Verification items for the finished model (mm, model axes). A direction names the side the tool comes from. Give positions to 0.01 mm unless a question says otherwise; leave off trailing zeros. Order: outer loops, then holes, each group sorted by start corner. A loop starts at its lowest first (then second) coordinate and runs counter-clockwise, first axis right, second up.
from build123d import *

# Parameters (mm, degrees)
BOSS_EXTRUDE2_DEPTH = 50.25
SKETCH3_W           = 2
SKETCH3_H           = 1
CUT_EXTRUDE2_DEPTH  = 101.5
SKETCH4_W           = 4
SKETCH4_H           = 2
BOSS_EXTRUDE3_DEPTH = 5
CUT_EXTRUDE3_DEPTH  = 5.2


with BuildPart() as part:
    # LED Segment → Boss-Extrude2 (new body, symmetric)
    with BuildSketch(Plane(origin=(0, 0, 0), x_dir=(0, 0, -1), z_dir=(1, 0, 0))):
        Polygon((8.982863896, -5.225833025), (12, 0), (6, 10.392304845), (-6, 10.392304845), (-12, 0), (-8.982863896, -5.225833025), (-4.7, 2.192304845), (-4.7, 2.792304845), (-6.1, 4.192304845), (-6.1, 4.792304845), (-5.1, 4.792304845), (-5.1, 5.392304845), (5.1, 5.392304845), (5.1, 4.792304845), (6.1, 4.792304845), (6.1, 4.192304845), (4.7, 2.792304845), (4.7, 2.192304845), align=None)
    extrude(amount=BOSS_EXTRUDE2_DEPTH, both=True)

    # Sketch3 → Cut-Extrude2 (cut, through all)
    with BuildSketch(Plane(origin=(50.25, 0, 0), x_dir=(0, 0, -1), z_dir=(1, 0, 0))):
        with Locations((4, 9.892304845)):
            Rectangle(SKETCH3_W, SKETCH3_H)
        Polygon((10.5, -2.598076211), (11.5, -0.866025404), (10.633974596, -0.366025404), (9.633974596, -2.098076211), align=None)
    extrude(amount=-CUT_EXTRUDE2_DEPTH, mode=Mode.SUBTRACT)

    # Sketch4 → Boss-Extrude3 (add)
    with BuildSketch(Plane(origin=(50.25, 0, 0), x_dir=(0, 0, -1), z_dir=(1, 0, 0))):
        with Locations((0, 9.392304845)):
            Rectangle(SKETCH4_W, SKETCH4_H)
    extrude(amount=BOSS_EXTRUDE3_DEPTH)

    # Sketch5 → Cut-Extrude3 (cut)
    with BuildSketch(Plane.ZY.offset(50.25)):
        Polygon((-2.2, 10.392304845), (-2.2, 8.192304845), (2.2, 8.192304845), (2.2, 10.392304845), (2, 10.392304845), (-2, 10.392304845), align=None)
    extrude(amount=-CUT_EXTRUDE3_DEPTH, mode=Mode.SUBTRACT)


solid = part.part
(1) Set-up check for faces 5 (the flat face through (53, 9, 2)), 6 (the flat face through (-48, 9, 2.2)), 7 (the flat face through (0.7, -1.46, -6.81)): record each of +Z, -Z, +X, -X, +Y, -Y from which the full face is reachable in a straight line by a thin tool's end or side.
Solved:
face 5: +Z, +X, +Y, -Y
face 6: -X, +Y
face 7: +X, -X, -Y
(2) Go/stop test with flat-tipped pins: pin 1 (1 mm diameter, centred on x = 39, y = -2, fed in from +Z); pin 2 (4 mm diameter, centred on y = 8.5, z = 8, fed in from +X); pin 3 (0.7 mm diameter, centred on x = -7, y = 4.5, fed in from -Z). Record where each tip stops, or that it passes through.
Solved:
pin 1: stops at z = 11.13
pin 2: stops at x = 50.25
pin 3: stops at z = -9.6
(3) Release check for a two-part mould opening along Y. For faces 1 (the flat face through (0.7, -1.22, -10.14)), 2 (the flat face through (0.7, -2.6, 10.5)), 3 (the flat face through (1, 9.392, -4)), 4 (the flat face through (-45.05, 9, 0)) record: pulls with the +Y half, pulls with the -Y half, needs draft (parallel to the pull), parting line crosses it, or undercut.
Solved:
face 1: undercut
face 2: pulls with the -Y half
face 3: pulls with the +Y half
face 4: needs draft
(4) Scan lines: line 1 (Z direction, x = 36.5, y = 1.25); line 2 (Z direction, x = -43.5, y = 9.5); line 3 (Y direction, x = -36, z = 1). Record each from-to range of solid material in increasing order.
Solved:
line 1: z = -11.28 to -5.24, 5.24 to 11.28
line 2: z = -6.52 to -5, -3 to 6.52
line 3: y = 5.39 to 10.39
(5) Section check A-A, the plane z = -0.25. Enter the section's corners in (x, y).
Solved:
outline: (-50.25, 5.39) - (50.25, 5.39) - (50.25, 8.39) - (55.25, 8.39) - (55.25, 10.39) - (-45.05, 10.39) - (-45.05, 8.19) - (-50.25, 8.19) - close
(6) Section check B-B, the plane x = -12. Enter the section's corners in (y, z).
Solved:
outline: (-5.23, -8.98) - (-2.6, -10.5) - (-2.1, -9.63) - (-0.37, -10.63) - (-0.87, -11.5) - (0, -12) - (10.39, -6) - (10.39, -5) - (9.39, -5) - (9.39, -3) - (10.39, -3) - (10.39, 6) - (0, 12) - (-5.23, 8.98) - (2.19, 4.7) - (2.79, 4.7) - (4.19, 6.1) - (4.79, 6.1) - (4.79, 5.1) - (5.39, 5.1) - (5.39, -5.1) - (4.79, -5.1) - (4.79, -6.1) - (4.19, -6.1) - (2.79, -4.7) - (2.19, -4.7) - close
